The drawing under review shows one solid part. Ordinate dimensions are in mm from its lowest x, y, z. A direction names the side the tool comes from. Round coordinates to 2 decimals unless told otherwise and drop trailing zeros. Order: outer loops, then holes, each group sorted by start corner. A loop starts at its lowest first (then second) coordinate and runs counter-clockwise, first axis right, second up. Notation, with made-up numbers: M -34.75,71.25 L -26.75,71.25 A34 ccw -26.75,102.25 Z; hole C -16,-19 d8. An arc over 180 degrees is marked long. Use a Markdown table: item, result.
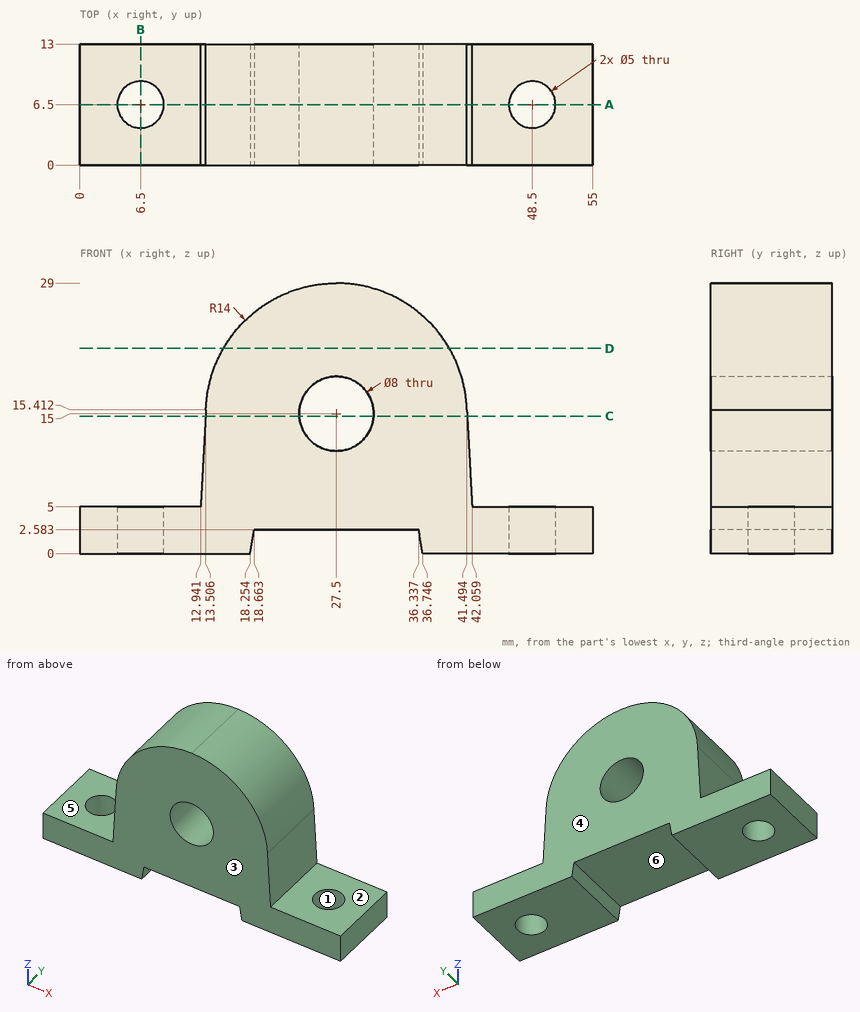
Q1. Draft analysis for pull direction Y (two halves, no side actions). For the marked faces 1, 2 and 3, state which applies: pulls with the +Y half, pulls with the -Y half, needs draft (parallel to the pull), parting line crosses it, or undercut.
Determined:
| item | result |
|---|---|
| face 1 | undercut |
| face 2 | needs draft |
| face 3 | pulls with the -Y half |
Q2. Clearance check with flat-ended pins moving along their axes: pin 1 (4 mm diameter, centred on x = 29.5, y = 7, fed in from -Z); pin 2 (12 mm diameter, centred on x = 35, z = 13.5, fed in from -Y); pin 3 (4 mm diameter, centred on y = 8.5, z = 23, fed in from +X); pin 4 (6 mm diameter, centred on y = 11, z = 12, fed in from +X). State where each tip first meets the part, or that it passes through.
Determined:
| item | result |
|---|---|
| pin 1 | stops at z = 2.58 |
| pin 2 | stops at y = 0 |
| pin 3 | stops at x = 40.15 |
| pin 4 | stops at x = 41.84 |
Q3. Add section D-D (z = 22). Write out the cut boundary in (x, y) (1 decimal).
Determined:
| item | result |
|---|---|
| outline | M 15.4,0 L 39.6,0 L 39.6,13 L 15.4,13 Z |
Q4. Add section C-C (z = 14.75). Write out the cut boundary in (x, y), then the cut area to 3 significant figures.
Determined:
| item | result |
|---|---|
| outline | M 13.47,0 L 23.51,0 L 23.51,13 L 13.47,13 Z; M 31.49,0 L 41.53,0 L 41.53,13 L 31.49,13 Z |
| area | 261 mm^2 |
Q5. Wall thickness on line 1 along X through (y, z) = (6.5, 3.3); line 2 along X through (y, z) = (8, 15); line 3 along Z through (x, y) = (3, 8.75): over which ranges is each line inside the solid? List them lowest first. Write a range as [from, to].
Determined:
| item | result |
|---|---|
| line 1 | x = [0, 4], [9, 46], [51, 55] |
| line 2 | x = [13.48, 23.5], [31.5, 41.52] |
| line 3 | z = [0, 5] |
Q6. Add section A-A (y = 6.5). Write out the cut boundary in (x, z).
Determined:
| item | result |
|---|---|
| outline | M 0,0 L 4,0 L 4,5 L 0,5 Z; M 9,0 L 18.25,0 L 18.66,2.58 L 36.34,2.58 L 36.75,0 L 46,0 L 46,5 L 42.06,5 L 41.49,15.41 A14 ccw 27.5,29 A14 ccw 13.51,15.41 L 12.94,5 L 9,5 Z; M 51,0 L 55,0 L 55,5 L 51,5 Z; hole C 27.5,15 d8 |
Q7. Machinability: for the marked faces 4, 5 and 6, which of the approach directions +Z, -Z, +X, -X, +Y, -Y give a long, thin tool a straight path to every point of the face, cutting with its end or side? Answer none if there is none.
Determined:
| item | result |
|---|---|
| face 4 | +Z, -Z, +X, -X, +Y |
| face 5 | +Z, -X, +Y, -Y |
| face 6 | -Z, +Y, -Y |
Q8. Add section B-B (x = 6.5). Write out the cut boundary in (y, z).
Determined:
| item | result |
|---|---|
| outline | M 0,0 L 4,0 L 4,5 L 0,5 Z; M 9,0 L 13,0 L 13,5 L 9,5 Z |
